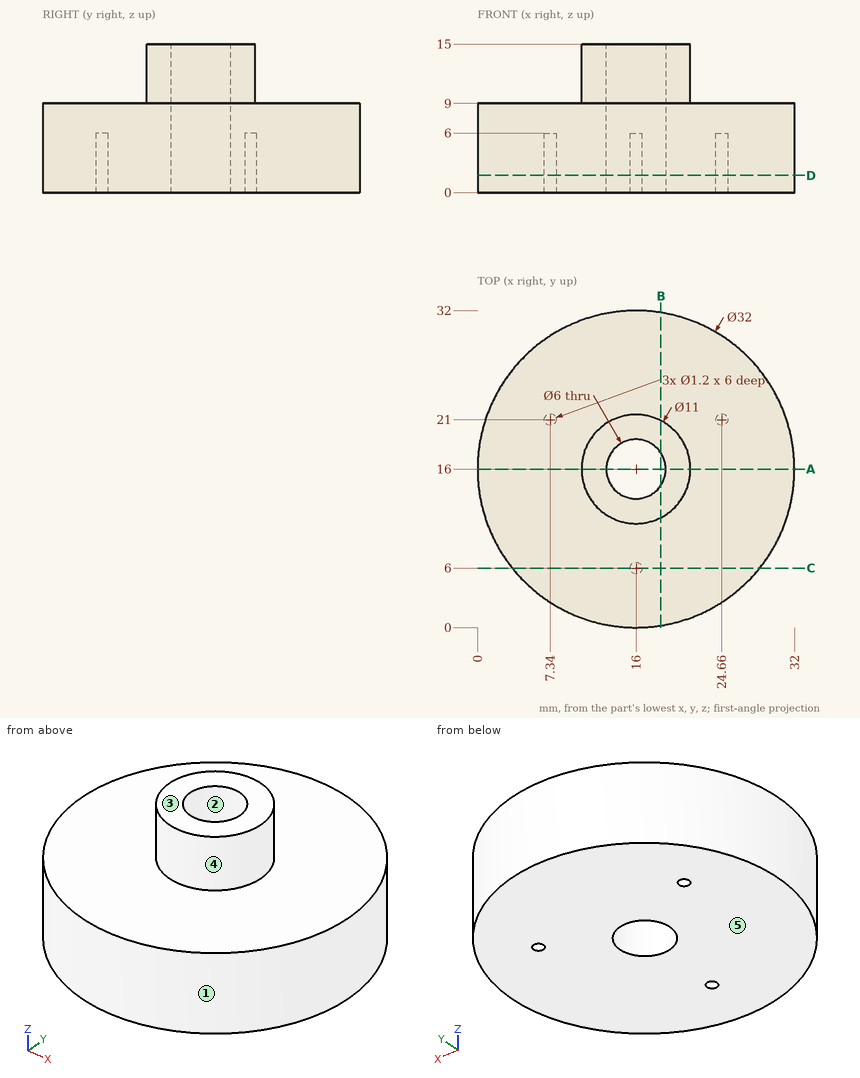
Job drawing, mm, ordinate dimensions from the low corner. One solid piece. A direction names the side the tool comes from. Give positions to 0.01 mm unless a question says otherwise; leave off trailing zeros. Write each loop counter-clockwise with the first axis right and the second up, starting at its lowest first coordinate (ties: lowest second). Pieces come first, ordered by that corner, then holes. Notation, with made-up numbers: M 72,44.25 L 104,44.25 A31 cw 104,72.25 Z; hole C -13.75,65 d9. An arc over 180 degrees is marked long. Put each result on its own line as item: value. Start each with the question number.
(1) Which spindle directions (+Z, -Z, +X, -X, +Y, -Y) get a long thin tool onto all of the face, cutting with end or side? Do the marked faces 4 and 5. Say none if no direction does.
(2) Band-saw the part on D-D, the plane z = 1.75. Write the cut outline in (x, y).
(3) Flat gauge pins, fed straight in: pin 1 Ø6 at (x, y) = (5.5, 8) entering from -Z; pin 2 Ø8 at (x, y) = (28, 21.5) entering from +Z; pin 3 Ø8 at (x, z) = (28, 4) entering from -Y; pin 4 Ø1.5 at (x, z) = (23, 8.5) entering from -Y. Where does each tip first touch, or does it go through?
(4) Probe L1, parallel to Y at x = 16, z = 4.7; L2, parallel to Y at x = 16, z = 10.5; L3, parallel to Y at x = 16, z = 7.5. List the from-to ranges inside material, lowest first.
(5) Band-saw the part on C-C, the plane y = 6. Write the cut outline in (x, z), and give its area (3 significant figures).
(6) Band-saw the part on A-A, the plane y = 16. Write the cut outline in (x, z).
(7) Band-saw the part on B-B, the plane x = 18.5. Write the cut outline in (y, z).
(8) Mould opens along Y. For the marked faces 1, 2 and 3 say: +Y half, -Y half, draft (parallel to the pull), parting line (faces both ways), or undercut.
Response values:
1. face 4: +Z
1. face 5: -Z, +X, -X, +Y, -Y
2. outline: C 16,16 d32; hole C 7.34,21 d1.2; hole C 16,16 d6; hole C 16,6 d1.2; hole C 24.66,21 d1.2
3. pin 1: stops at z = 0
3. pin 2: stops at z = 9
3. pin 3: stops at y = 2.14
3. pin 4: stops at y = 1.27
4. L1: y = 0 to 5.4, 6.6 to 13, 19 to 32
4. L2: y = 10.5 to 13, 19 to 21.5
4. L3: y = 0 to 13, 19 to 32
5. outline: M 3.51,0 L 15.4,0 L 15.4,6 L 16.6,6 L 16.6,0 L 28.49,0 L 28.49,9 L 3.51,9 Z
5. area: 218 mm2
6. outline: M 0,0 L 13,0 L 13,15 L 10.5,15 L 10.5,9 L 0,9 Z; M 19,0 L 32,0 L 32,9 L 21.5,9 L 21.5,15 L 19,15 Z
7. outline: M 0.2,0 L 14.34,0 L 14.34,15 L 11.1,15 L 11.1,9 L 0.2,9 Z; M 17.66,0 L 31.8,0 L 31.8,9 L 20.9,9 L 20.9,15 L 17.66,15 Z
8. face 1: parting line
8. face 2: undercut
8. face 3: draft
